```python
from build123d import *

# Parameters (mm, degrees)
SKETCH1_R           = 12
BOSS_EXTRUDE1_DEPTH = 3
SKETCH2_R           = 9.75
BOSS_EXTRUDE2_DEPTH = 7
SKETCH3_R           = 2.35
CUT_EXTRUDE1_DEPTH  = 5


with BuildPart() as part:
    # Sketch1 → Boss-Extrude1 (new body)
    with BuildSketch(Plane.XY):
        with Locations((-127.992538975, 40.103259291)):
            Circle(SKETCH1_R)
    extrude(amount=BOSS_EXTRUDE1_DEPTH)

    # Sketch2 → Boss-Extrude2 (add)
    with BuildSketch(Plane(origin=(0, 0, 0), x_dir=(-1, 0, 0), z_dir=(0, 0, -1))):
        with Locations((127.992538975, 40.103259291)):
            Circle(SKETCH2_R)
    extrude(amount=BOSS_EXTRUDE2_DEPTH)

    # Sketch3 → Cut-Extrude1 (cut)
    with BuildSketch(Plane(origin=(0, 0, -7), x_dir=(-1, 0, 0), z_dir=(0, 0, -1))):
        with Locations((127.992538975, 40.103259291)):
            Circle(SKETCH3_R)
    extrude(amount=-CUT_EXTRUDE1_DEPTH, mode=Mode.SUBTRACT)


solid = part.part
```
Work out the finished part from the listing and answer in its coordinate system (mm). A direction names the side the tool comes from. Coordinates: 2 decimals unless noted, no trailing zeros. Order: outer loops, then holes, each group sorted by start corner. A loop starts at its lowest first (then second) coordinate and runs counter-clockwise, first axis right, second up. Notation, with made-up numbers: (59, 30.5) - (83, 30.5) arc R15 ccw to (83, 59.5) - close; hole circle Ø11 at (-21.5, 56). An arc over 180 degrees is marked (long way). Answer as a JSON object with one key per item and string values.
1. Find section B-B on x = -120. Determine the outline of the cut face in (y, z).
Output values:
{"outline": "(31.15, 0) - (34.52, 0) - (34.52, -7) - (45.69, -7) - (45.69, 0) - (49.05, 0) - (49.05, 3) - (31.15, 3) - close"}
2. Find section A-A on y = 33.5. Determine the outline of the cut face in (x, z).
Output values:
{"outline": "(-138.01, 0) - (-135.17, 0) - (-135.17, -7) - (-120.82, -7) - (-120.82, 0) - (-117.97, 0) - (-117.97, 3) - (-138.01, 3) - close"}
3. Consider line 1 (X direction, y = 40, z = -0.25); line 2 (Z direction, x = -118.5, y = 35.5); line 3 (Y direction, x = -128.25, z = -3.75). Determine where each line is inside the solid, lowest interval first.
Output values:
{"line 1": "x = -137.74 to -118.24", "line 2": "z = 0 to 3", "line 3": "y = 30.36 to 37.77, 42.44 to 49.85"}
4. Find section C-C on z = -3.5. Determine the outline of the cut face in (x, y).
Output values:
{"outline": "circle Ø19.5 at (-127.99, 40.1); hole circle Ø4.7 at (-127.99, 40.1)"}
5. Each of these flat-tipped pins is pushed along its axis until it touches: P1, Ø3, axis at y = 31, z = 1, coming from the -X side; P2, Ø2, axis at x = -120, z = -1.5, coming from the -Y side; P3, Ø1.5, axis at x = -133.5, z = -5, coming from the -Y side. Where does it stop, or does it pass through?
Output values:
{"P1": "stops at x = -137.28", "P2": "stops at y = 33.31", "P3": "stops at y = 31.59"}
6. The mould has two halves that part along X. Classify faces 3 (the face through (-136.84, 48.21, 1.48)), 4 (the face through (-128, 40, -2)), 5 (the face through (-129, 50, 0)): +X half, -X half, draft (parallel to the pull), parting line (faces both ways), or undercut.
Output values:
{"face 3": "parting line", "face 4": "undercut", "face 5": "draft"}
7. Find section D-D on x = -129.5. Determine the outline of the cut face in (y, z).
Output values:
{"outline": "(28.2, 0) - (30.47, 0) - (30.47, -7) - (38.3, -7) - (38.3, -2) - (41.91, -2) - (41.91, -7) - (49.74, -7) - (49.74, 0) - (52.01, 0) - (52.01, 3) - (28.2, 3) - close"}
8. A tool of negligible diameter and unlimited length cuts with its end or side. For faces 1 (the face through (-130, 38, -7)), 2 (the face through (-125.645, 40.207, -4.535)), from which of +Z, -Z, +X, -X, +Y, -Y can it reach the whole face along a straight path? Write none if from no direction.
Output values:
{"face 1": "-Z, +X, -X, +Y, -Y", "face 2": "-Z"}
